The drawing under review shows one solid part. Ordinate dimensions are in mm from its lowest x, y, z. A direction names the side the tool comes from. Round coordinates to 2 decimals unless told otherwise and drop trailing zeros. Order: outer loops, then holes, each group sorted by start corner. A loop starts at its lowest first (then second) coordinate and runs counter-clockwise, first axis right, second up. Notation, with made-up numbers: M -2.75,78 L 30.25,78 A18 cw 30.25,96 Z; hole C -15.5,71.5 d7. An arc over 180 degrees is marked long. Answer as a JSON object with one key per item and string values. Group by question number.
1. Clearance check with flat-ended pins moving along their axes: P1, Ø10, axis at x = 346, y = 87.5, coming from the -Z side; P2, Ø10, axis at y = 187, z = 110, coming from the -X side. State where each tip first meets the part, or that it passes through.
2. Add section A-A on z = 184.5. State the section outline as (x, y) points, and give its area (3 significant figures).
3. Machinability: for the marked faces 5 and 6, which of the approach directions +Z, -Z, +X, -X, +Y, -Y give a long, thin tool a straight path to every point of the face, cutting with its end or side? Answer none if there is none.
4. Add section B-B on x = 595. State the section outline as (y, z) points, and give its area (3 significant figures).
5. Add section C-C on y = 39. State the section outline as (x, z) points, and give its area (3 significant figures).
6. To check wall thickness, follow probe 1 along X at (y, z) = (220, 260); probe 2 along Z at (x, y) = (208, 102.5). State the ranges of each line that lie inside material, in increasing order. Write a range as [from, to].
7. Mouldability with a two-part tool opening along X and no side actions: class the marked faces 1, 2, 3 and 4 as released by +X, released by -X, zero draft, split by the parting line, or undercut.
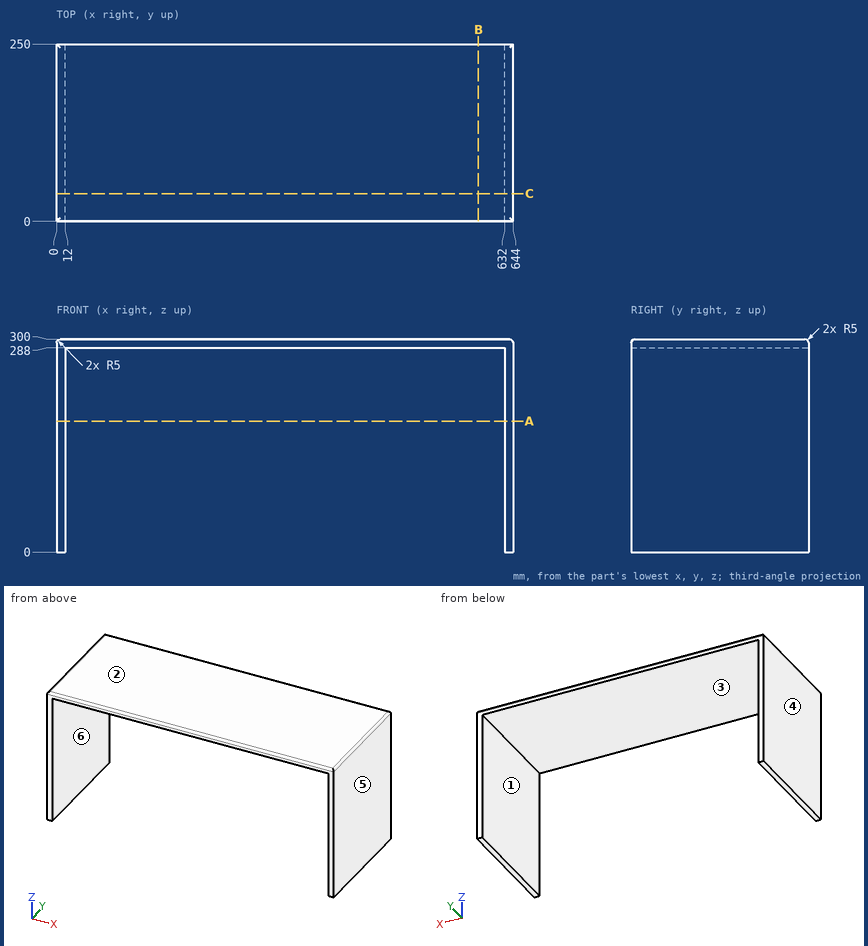
Recorded:
{
 "1": {"P1": "stops at z = 288", "P2": "stops at x = 0"},
 "2": {"outline": "M 0,0 L 12,0 L 12,250 L 0,250 Z; M 632,0 L 644,0 L 644,250 L 632,250 Z", "area": "6,000 mm²"},
 "3": {"face 5": "+Z, -Z, +X, +Y, -Y", "face 6": "-Z, +Y, -Y"},
 "4": {"outline": "M 0,288 L 250,288 L 250,295 A5 ccw 245,300 L 5,300 A5 ccw 0,295 Z", "area": "2,990 mm²"},
 "5": {"outline": "M 0,0 L 12,0 L 12,288 L 632,288 L 632,0 L 644,0 L 644,295 A5 ccw 639,300 L 5,300 A5 ccw 0,295 Z", "area": "14,600 mm²"},
 "6": {"probe 1": "x = [0, 12], [632, 644]", "probe 2": "z = [288, 300]"},
 "7": {"face 1": "undercut", "face 2": "zero draft", "face 3": "undercut", "face 4": "released by -X"}
}
